Build history of the part. All positions in model axes, mm. A direction names the side the tool comes from. Round coordinates to 2 decimals unless told otherwise and drop trailing zeros. Loops run counter-clockwise (first coordinate to the right, second up) from the corner with the lowest first, then second, coordinate; pieces in that order, holes last. Notation, with made-up numbers: (69.25, -28.5) - (102.25, -28.5) arc R22 cw to (102.25, -16.5) - close; hole circle Ø8 at (86, -40). An arc over 180 degrees is marked (long way). Answer as CSV lines item,"result". Start each with the question number.
```python
from build123d import *

# Parameters (mm, degrees)
F0_R     = 12.7
F1_DEPTH = 38.1
F2_R     = 1.651
F3_DEPTH = 12.7


with BuildPart() as f1:
    # F0 (on Right) → F1 (new body, symmetric)
    with BuildSketch(Plane.YZ):
        with BuildLine():
            Line((19.05, -29.424714), (19.05, 0))
            ThreePointArc((19.05, 0), (0, 19.05), (-19.05, 0))
            Line((-19.05, 0), (-19.05, -29.424714))
            Line((-19.05, -29.424714), (19.05, -29.424714))
        make_face()
        Circle(F0_R, mode=Mode.SUBTRACT)
    extrude(amount=F1_DEPTH, both=True)

    # F2 (on face) → F3 (cut)
    with BuildSketch(Plane(origin=(0, 0, -29.424714), x_dir=(1, 0, 0), z_dir=(0, 0, -1))):
        with Locations((31.75, 12.7)):
            Circle(F2_R)
        with Locations((-31.75, 12.7)):
            Circle(F2_R)
        with Locations((-31.75, -12.7)):
            Circle(F2_R)
        with Locations((31.75, -12.7)):
            Circle(F2_R)
    extrude(amount=-F3_DEPTH, mode=Mode.SUBTRACT)


solid = f1.part
```
Q1. Tool access for faces 5 (the flat face through (1, 0, -29.425)), 6 (the cylindrical face through (32.512, 14.165, -23.164)): list every direction of +Z, -Z, +X, -X, +Y, -Y with a clear straight run to the whole face (end or side of a thin tool).
Q2. Two-plate mould, pull along X, no slides. Class faces 1 (the cylindrical face through (0.533, 0.419, 19.045)), 2 (the flat face through (-32, -13, -16.725)), 3 (the flat face through (38.1, 0, -16)), 4 (the flat face through (-38.1, 0, -16)): released by +X, released by -X, zero draft, split by the parting line, or undercut.
Q3. Band-saw the part on D-D, the plane x = 12. List the corners of the cut face in (y, z), then the cut area to 3 significant figures.
Q4. Band-saw the part on C-C, the plane x = 31.75. List the corners of the cut face in (y, z).
Q5. Band-saw the part on A-A, the plane y = 0. List the corners of the cut face in (x, z).
Q6. Pin check, flat tips, straight feed: pin 1 Ø1.7 at (x, y) = (31.5, -13) entering from -Z; pin 2 Ø6 at (x, y) = (-4.5, 9) entering from +Z; pin 3 Ø6 at (y, z) = (-7, -6.5) entering from -X; pin 4 Ø1.5 at (x, z) = (-23, 12.5) entering from +Y. Stop position of each tip, or through.
Q7. Wall check: probe 1 along X at (y, z) = (12.7, -21.75); probe 2 along Y at (x, z) = (-31.75, -19.5); probe 3 along Z at (x, y) = (19, 0). Give the ranges that are in metal, low to high. Write a range as [from, to].
Q8. Band-saw the part on B-B, the plane z = 10.5. List the corners of the cut face in (x, y).
Reported:
1,face 5,"-Z, +X, -X, +Y, -Y"
1,face 6,"-Z"
2,face 1,"zero draft"
2,face 2,"undercut"
2,face 3,"released by +X"
2,face 4,"released by -X"
3,outline,"(-19.05, -29.42) - (19.05, -29.42) - (19.05, 0) arc R19.05 ccw to (-19.05, 0) - close; hole circle Ø25.4 at (0, 0)"
3,area,"1,180 mm2"
4,outline,"(-19.05, -29.42) - (-14.35, -29.42) - (-14.35, -16.72) - (-11.05, -16.72) - (-11.05, -29.42) - (11.05, -29.42) - (11.05, -16.72) - (14.35, -16.72) - (14.35, -29.42) - (19.05, -29.42) - (19.05, 0) arc R19.05 ccw to (-19.05, 0) - close; hole circle Ø25.4 at (0, 0)"
5,outline,"(-38.1, -29.42) - (38.1, -29.42) - (38.1, -12.7) - (-38.1, -12.7) - close; (-38.1, 12.7) - (38.1, 12.7) - (38.1, 19.05) - (-38.1, 19.05) - close"
6,pin 1,"stops at z = -16.72"
6,pin 2,"stops at z = 18.08"
6,pin 3,"passes through"
6,pin 4,"stops at y = 14.99"
7,probe 1,"x = [-38.1, -33.4], [-30.1, 30.1], [33.4, 38.1]"
7,probe 2,"y = [-19.05, -14.35], [-11.05, 11.05], [14.35, 19.05]"
7,probe 3,"z = [-29.42, -12.7], [12.7, 19.05]"
8,outline,"(-38.1, -15.9) - (38.1, -15.9) - (38.1, -7.14) - (-38.1, -7.14) - close; (-38.1, 7.14) - (38.1, 7.14) - (38.1, 15.9) - (-38.1, 15.9) - close"
